```python
from build123d import *


with BuildPart() as part:
    # Esquisse1 → Révolution1 (revolve)
    with BuildSketch(Plane.XY):
        with BuildLine():
            Line((0, 3), (1, 3))
            Line((1, 3), (1, 2))
            Line((1, 2), (11.845299462, 2))
            Line((11.845299462, 2), (13, 0))
            Line((13, 0), (1.154700538, 0))
            Line((1.154700538, 0), (0, 2))
            Line((0, 2), (-0.5, 2))
            ThreePointArc((-0.5, 2), (-0.853553391, 2.146446609), (-1, 2.5))
            Line((-1, 2.5), (-1, 3.5))
            ThreePointArc((-1, 3.5), (-0.853553391, 3.853553391), (-0.5, 4))
            Line((-0.5, 4), (0, 4))
            Line((0, 4), (0, 3))
        make_face()
    revolve(axis=Axis((-8.537570942, 0, 0), (1, 0, 0)))


solid = part.part
```
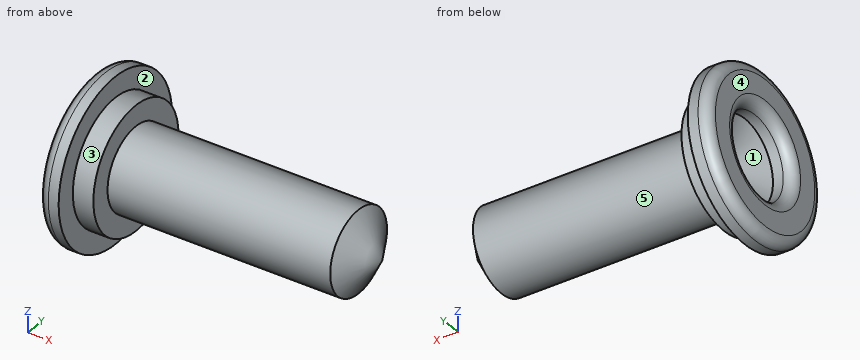
The model under review builds one solid part; all positions refer to its coordinate system, in mm. Face numbers are marked on the shaded views. A direction names the side the tool comes from. Round coordinates to 2 decimals unless told otherwise and drop trailing zeros. Loops run counter-clockwise (first coordinate to the right, second up) from the corner with the lowest first, then second, coordinate; pieces in that order, holes last. Notation, with made-up numbers: (-16.75, 38) - (-12.75, 38) arc R18 ccw to (-12.75, 57) - close; hole circle Ø4 at (38.5, 6). An arc over 180 degrees is marked (long way). Write each question's results on one line, items separated by ' | '. Start each with the question number.
Q1. Insertion check: P1, Ø1, axis at x = 9, z = -2, coming from the +Y side; P2, Ø1, axis at x = 8, y = -2, coming from the +Z side; P3, Ø4, axis at x = 3, z = 3, coming from the -Y side. Each pin has a flat end and moves straight along its axis. Give the tip position at first contact, or say it passes through.
Q2. Tool access review of the marked faces 4 and 5: name each direction out of +Z, -Z, +X, -X, +Y, -Y from which nothing blocks a thin tool from reaching the whole face with its end or side.
Q3. Wall thickness on line 1 along Z through (x, y) = (-0.15, 0); line 2 along X through (y, z) = (-3, 1.25); line 3 along Z through (x, y) = (0.75, -0.25): over which ranges is each line inside the solid? List them lowest first. Write a range as [from, to].
Q4. Take a section at B-B on x = 0.75. Give the boundary of the cut face in (y, z), plus the area to 3 significant figures.
Q5. Take a section at A-A on x = 5.25. Give the boundary of the cut face in (y, z).
Q6. Draft analysis for pull direction Z (two halves, no side actions). For the marked faces 1, 2 and 3, state which applies: pulls with the +Z half, pulls with the -Z half, needs draft (parallel to the pull), parting line crosses it, or undercut.
Data:
1) P1: stops at y = 1.32 | P2: stops at z = 1.32 | P3: stops at y = -1.73
2) face 4: +Z, -Z, -X, +Y, -Y | face 5: +X
3) line 1: z = [-4, -2], [2, 4] | line 2: x = [-1, 0] | line 3: z = [-2.99, -0.65], [0.65, 2.99]
4) outline: circle Ø6 at (0, 0); hole circle Ø1.4 at (0, 0) | area: 26.7 mm²
5) outline: circle Ø4 at (0, 0)
6) face 1: undercut | face 2: needs draft | face 3: parting line crosses it
